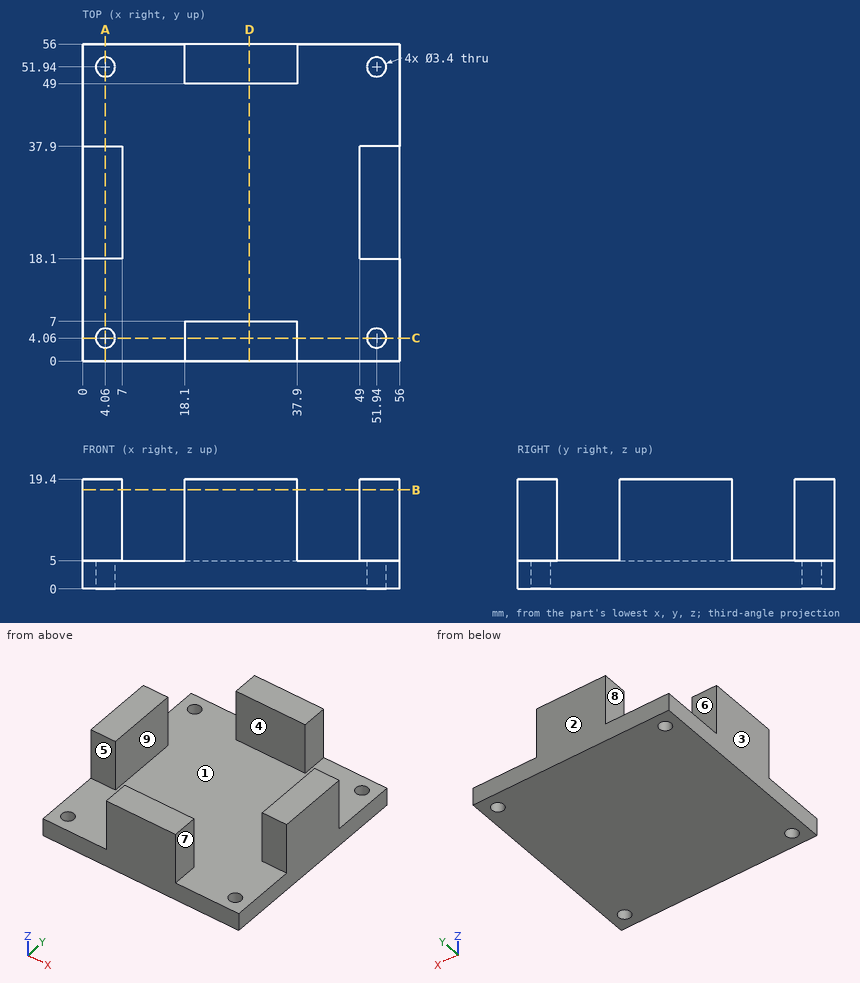
For this review, use the dimensioned drawing (mm, ordinates from the lowest corner) and the shaded views. A direction names the side the tool comes from. Give positions to 0.01 mm unless a question says otherwise; leave off trailing zeros. Write each loop counter-clockwise with the first axis right and the second up, starting at its lowest first coordinate (ties: lowest second). Pieces come first, ordered by that corner, then holes. Notation, with made-up numbers: M 89.5,-10.75 L 115.5,-10.75 A20 cw 115.5,18.25 Z; hole C 88.5,17 d10. An arc over 180 degrees is marked long. Answer as a JSON object with one key per item and string values. Group by question number.
Item 1: Consider section D-D on x = 29.5. Write out the cut boundary in (y, z), plus the area to 3 significant figures.
Item 2: Draft analysis for pull direction Y (two halves, no side actions). For the marked faces 1, 2, 3 and 4, state which applies: +Y half, -Y half, draft (parallel to the pull), parting line (faces both ways), or undercut.
Item 3: Consider section B-B on z = 17.5. Write out the cut boundary in (x, y).
Item 4: Consider section A-A on x = 4.06. Write out the cut boundary in (y, z), plus the area to 3 significant figures.
Item 5: For probe 1 along Y at (x, z) = (51.94, 2.2); probe 2 along X at (y, z) = (23, 6.25), list the stretches that pass through material, from the lowest coordinate up. Write a range as [from, to].
Item 6: Tool access review of the marked faces 5, 6, 7, 8 and 9: name each direction out of +Z, -Z, +X, -X, +Y, -Y from which nothing blocks a thin tool from reaching the whole face with its end or side.
Item 7: For pin 1 Ø4 at (x, y) = (33.5, 16.5) entering from +Z; pin 2 Ø5.5 at (x, z) = (51, 13.5) entering from +Y; pin 3 Ø7.5 at (y, z) = (51, 11) entering from -X, all flat-tipped, find the tip position at first contact; note any pin that passes through.
Check result:
{
 "1": {"outline": "M 0,0 L 56,0 L 56,19.4 L 49,19.4 L 49,5 L 7,5 L 7,19.4 L 0,19.4 Z", "area": "482 mm^2"},
 "2": {"face 1": "undercut", "face 2": "+Y half", "face 3": "draft", "face 4": "undercut"},
 "3": {"outline": "M 0,18.1 L 7,18.1 L 7,37.9 L 0,37.9 Z; M 18.1,0 L 37.9,0 L 37.9,7 L 18.1,7 Z; M 18.1,49 L 37.9,49 L 37.9,56 L 18.1,56 Z; M 49,18.1 L 56,18.1 L 56,37.9 L 49,37.9 Z"},
 "4": {"outline": "M 0,0 L 2.36,0 L 2.36,5 L 0,5 Z; M 5.76,0 L 50.24,0 L 50.24,5 L 37.9,5 L 37.9,19.4 L 18.1,19.4 L 18.1,5 L 5.76,5 Z; M 53.64,0 L 56,0 L 56,5 L 53.64,5 Z", "area": "531 mm^2"},
 "5": {"probe 1": "y = [0, 2.36], [5.76, 50.24], [53.64, 56]", "probe 2": "x = [0, 7], [49, 56]"},
 "6": {"face 5": "+Z, +X, -X, -Y", "face 6": "+Z, +X, -X, +Y", "face 7": "+Z, +X, +Y, -Y", "face 8": "+Z, -X, +Y, -Y", "face 9": "+Z, +Y, -Y"},
 "7": {"pin 1": "stops at z = 5", "pin 2": "stops at y = 37.9", "pin 3": "stops at x = 18.1"}
}
